Input: part model. Units: mm. Frame: model coordinates. Face numbers are marked on the shaded views. A direction names the side the tool comes from. Give positions to 0.01 mm unless a question says otherwise; leave off trailing zeros. Loops run counter-clockwise (first coordinate to the right, second up) from the corner with the lowest first, then second, coordinate; pieces in that order, holes last. Notation, with made-up numbers: (84.5, -7.75) - (102.5, -7.75) arc R35 cw to (102.5, 24.25) - close; hole circle Ø8 at (51.5, 7.25). An arc over 180 degrees is marked (long way). One line per item, written item: value.
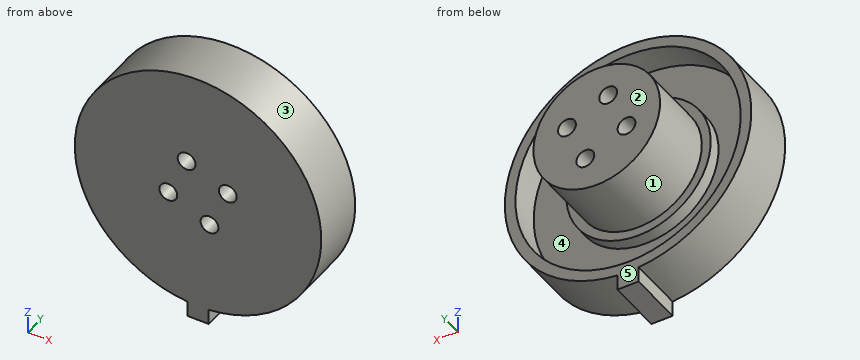
from build123d import *

# Parameters (mm, degrees)
SKETCH1_R           = 29
BOSS_EXTRUDE1_DEPTH = 13
SKETCH2_R           = 26.5
SKETCH2_R_2         = 17
CUT_EXTRUDE1_DEPTH  = 7
SKETCH4_R           = 17.25
CUT_EXTRUDE3_DEPTH  = 4
SKETCH5_W           = 5
SKETCH5_H           = 4.624873007
BOSS_EXTRUDE2_DEPTH = 13
SKETCH6_R           = 14.9
BOSS_EXTRUDE3_DEPTH = 16
SKETCH3_R           = 2.1
CUT_EXTRUDE2_DEPTH  = 30


with BuildPart() as part:
    # Sketch1 → Boss-Extrude1 (new body)
    with BuildSketch(Plane(origin=(0, 0, 0), x_dir=(1, 0, 0), z_dir=(0, 1, 0))):
        with Locations(Location((0, 0, 0), (0, 0, 90))):
            Circle(SKETCH1_R)
    extrude(amount=BOSS_EXTRUDE1_DEPTH)

    # Sketch2 → Cut-Extrude1 (cut)
    with BuildSketch(Plane(origin=(0, 13, 0), x_dir=(1, 0, 0), z_dir=(0, 1, 0))):
        with Locations(Location((0, 0, 0), (0, 0, 270))):
            Circle(SKETCH2_R)
        with Locations(Location((0, 0, 0), (0, 0, 270))):
            Circle(SKETCH2_R_2, mode=Mode.SUBTRACT)
    extrude(amount=-CUT_EXTRUDE1_DEPTH, mode=Mode.SUBTRACT)

    # Sketch4 → Cut-Extrude3 (cut)
    with BuildSketch(Plane(origin=(0, 13, 0), x_dir=(1, 0, 0), z_dir=(0, 1, 0))):
        Circle(SKETCH4_R)
    extrude(amount=-CUT_EXTRUDE3_DEPTH, mode=Mode.SUBTRACT)

    # Sketch5 → Boss-Extrude2 (add)
    with BuildSketch(Plane.XZ):
        with Locations((0, -30.234113057)):
            Rectangle(SKETCH5_W, SKETCH5_H)
    extrude(amount=-BOSS_EXTRUDE2_DEPTH)

    # Sketch6 → Boss-Extrude3 (add)
    with BuildSketch(Plane(origin=(0, 9, 0), x_dir=(1, 0, 0), z_dir=(0, 1, 0))):
        with Locations(Location((0, 0, 0), (0, 0, 270))):
            Circle(SKETCH6_R)
    extrude(amount=BOSS_EXTRUDE3_DEPTH)

    # Sketch3 → Cut-Extrude2 (cut)
    with BuildSketch(Plane.XZ):
        with Locations(Location((7.002624358, 2.68574982, 0), (0, 0, 270))):
            Circle(SKETCH3_R)
        with Locations(Location((-7.002624358, -2.68574982, 0), (0, 0, 270))):
            Circle(SKETCH3_R)
        with Locations(Location((2.68574982, -7.002624358, 0), (0, 0, 270))):
            Circle(SKETCH3_R)
        with Locations(Location((-2.68574982, 7.002624358, 0), (0, 0, 270))):
            Circle(SKETCH3_R)
    extrude(amount=-CUT_EXTRUDE2_DEPTH, mode=Mode.SUBTRACT)


solid = part.part
Item 1: Access query for the marked faces 1 and 2. Directions: +Z, -Z, +X, -X, +Y, -Y. A direction counts if a zero-diameter tool reaches every point of the face in a straight line with its end or side. Return the directions, or none.
Verdict:
face 1: +Y
face 2: +Z, -Z, +X, -X, +Y
Item 2: Section D-D, the plane x = 24. Output: boundary loops of the cut face in (y, z), and give its area (3 significant figures).
Verdict:
outline: (0, -16.28) - (13, -16.28) - (13, -11.24) - (6, -11.24) - (6, 11.24) - (13, 11.24) - (13, 16.28) - (0, 16.28) - close
area: 266 mm^2
Item 3: Section C-C, the plane y = 4.5. Output: boundary loops of the cut face in (x, z).
Verdict:
outline: (-2.5, -32.55) - (2.5, -32.55) - (2.5, -28.89) arc R29 ccw (long way) to (-2.5, -28.89) - close; hole circle Ø4.2 at (-7, -2.69); hole circle Ø4.2 at (-2.69, 7); hole circle Ø4.2 at (2.69, -7); hole circle Ø4.2 at (7, 2.69)
Item 4: Pin query (flat end, axial travel): P1, Ø2, axis at y = 13.5, z = -6.5, coming from the +X side; P2, Ø1.5, axis at y = 11, z = 22.5, coming from the -X side; P3, Ø12, axis at y = 19.5, z = -22, coming from the -X side; P4, Ø12, axis at x = -10.5, y = 6.5, coming from the -Z side. Return the tip coordinate at first contact, or that it passes through.
Verdict:
P1: stops at x = 28.45
P2: stops at x = -19.18
P3: passes through
P4: stops at z = -28.65
Item 5: Draft query along X for the marked faces 3, 4 and 5. Return one class per face: pulls with the +X half, pulls with the -X half, needs draft (parallel to the pull), parting line crosses it, or undercut.
Verdict:
face 3: parting line crosses it
face 4: undercut
face 5: needs draft
Item 6: Section A-A, the plane y = 11.25. Output: boundary loops of the cut face in (x, z), and give its area (3 significant figures).
Verdict:
outline: circle Ø29.8 at (0, 0); (-2.5, -32.55) - (2.5, -32.55) - (2.5, -28.89) arc R29 ccw (long way) to (-2.5, -28.89) - close; hole circle Ø53 at (0, 0); hole circle Ø4.2 at (-7, -2.69); hole circle Ø4.2 at (-2.69, 7); hole circle Ø4.2 at (2.69, -7); hole circle Ø4.2 at (7, 2.69)
area: 1,100 mm^2
Item 7: Material intervals for L1, parallel to X at y = 8.75, z = 0; L2, parallel to X at y = 10.25, z = 0; L3, parallel to Z at x = -0.5, y = 8, sorted ascending.
Verdict:
L1: x = -29 to -26.5, -17 to 17, 26.5 to 29
L2: x = -29 to -26.5, -14.9 to 14.9, 26.5 to 29
L3: z = -32.55 to -26.5, -16.99 to 16.99, 26.5 to 29
Item 8: Section B-B, the plane z = 7. Output: boundary loops of the cut face in (x, y).
Verdict:
outline: (-28.14, 0) - (-4.79, 0) - (-4.79, 25) - (-13.15, 25) - (-13.15, 9) - (-15.49, 9) - (-15.49, 6) - (-25.56, 6) - (-25.56, 13) - (-28.14, 13) - close; (-0.59, 0) - (28.14, 0) - (28.14, 13) - (25.56, 13) - (25.56, 6) - (15.49, 6) - (15.49, 9) - (13.15, 9) - (13.15, 25) - (-0.59, 25) - close
